```python
from build123d import *

# Parameters (mm, degrees)
F0_W     = 30.48
F0_H     = 28
F1_DEPTH = 1
F3_W     = 30.48
F3_H     = 4.265539
F4_DEPTH = 0.5
F2_R     = 0.9
F2_R_2   = 0.7
F2_R_3   = 0.65
F5_DEPTH = 2


with BuildPart() as f1:
    # F0 (on Top) → F1 (new body)
    with BuildSketch(Plane.XY):
        Rectangle(F0_W, F0_H)
    extrude(amount=F1_DEPTH)

    # F3 (on face) → F4 (cut)
    with BuildSketch(Plane.XY.offset(1)):
        with Locations((0, 1.480549)):
            Rectangle(F3_W, F3_H)
    extrude(amount=-F4_DEPTH, mode=Mode.SUBTRACT)

    # F2 (on face) → F5 (cut)
    with BuildSketch(Plane.XY.offset(1)):
        with Locations((-11.36, 11.94)):
            Circle(F2_R)
        with Locations((-6.28, 11.94)):
            Circle(F2_R)
        with Locations((-1.2, 11.94)):
            Circle(F2_R)
        with Locations((8.96, 11.94)):
            Circle(F2_R)
        with Locations((14.04, 11.94)):
            Circle(F2_R)
        with Locations((-11.36, 6.86)):
            Circle(F2_R)
        with Locations((-6.28, 6.86)):
            Circle(F2_R)
        with Locations((-1.2, 6.86)):
            Circle(F2_R)
        with Locations((8.96, 6.86)):
            Circle(F2_R)
        with Locations((14.04, 6.86)):
            Circle(F2_R)
        with Locations((-11.36, -9.52)):
            Circle(F2_R_2)
        with Locations((-6.28, -9.52)):
            Circle(F2_R_2)
        with Locations((-1.2, -9.52)):
            Circle(F2_R_2)
        with Locations((8.96, -9.52)):
            Circle(F2_R_2)
        with Locations((14.04, -9.52)):
            Circle(F2_R_2)
        with Locations((-11.36, -13.3)):
            Circle(F2_R_3)
        with Locations((-6.28, -13.3)):
            Circle(F2_R_3)
        with Locations((-1.2, -13.3)):
            Circle(F2_R_3)
        with Locations((8.96, -13.3)):
            Circle(F2_R_3)
        with Locations((14.04, -13.3)):
            Circle(F2_R_3)
    extrude(amount=-F5_DEPTH, mode=Mode.SUBTRACT)


solid = f1.part
```
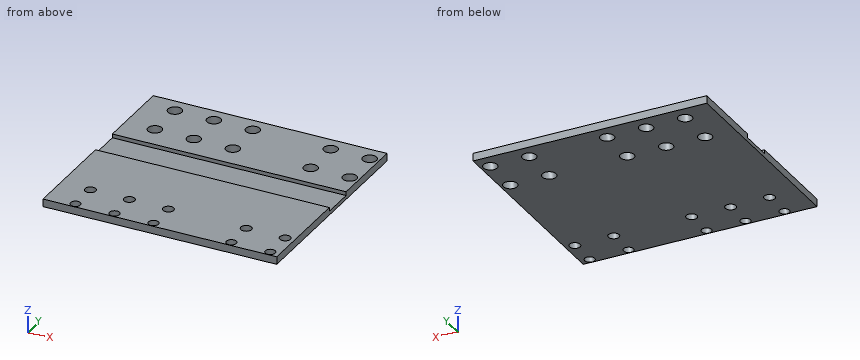
Geometry: final body of the model. Coordinates: model frame, mm. Coordinates: 2 decimals unless noted, no trailing zeros. Loops run counter-clockwise (first coordinate to the right, second up) from the corner with the lowest first, then second, coordinate; pieces in that order, holes last. Notation, with made-up numbers: (-23.5, 34) -> (9.5, 34) arc R22 ccw to (9.5, 45) -> close; hole circle Ø6 at (-6.5, 54). An arc over 180 degrees is marked (long way). Use a Markdown table: item, result. Add a question column.
(1) Section query C-C, the plane z = 0.8. State how many separate pieces and enclosed holes the cut face has, plus the area to 3 significant figures.
(2) Section query A-A, the plane x = -6.28. Return loops of the section in (y, z).
(3) Section query B-B, the plane y = -9.52. Return loops of the section in (x, z), plus the area to 3 significant figures.
(4) Line query: line 1 along X through (y, z) = (6.75, 0.15); line 2 along Z through (x, y) = (-7.5, 3.5); line 3 along X through (y, z) = (6.5, 0.9). Output: solid intervals per line, ascending.
(5) Section query D-D, the plane y = 6.86. Return loops of the section in (x, z).
Answer:
| question | item | result |
|---|---|---|
| 1 | separate pieces | 2 |
| 1 | enclosed holes | 20 |
| 1 | area | 684 mm^2 |
| 2 | outline | (-14, 0) -> (-13.95, 0) -> (-13.95, 1) -> (-14, 1) -> close; (-12.65, 0) -> (-10.22, 0) -> (-10.22, 1) -> (-12.65, 1) -> close; (-8.82, 0) -> (5.96, 0) -> (5.96, 1) -> (3.61, 1) -> (3.61, 0.5) -> (-0.65, 0.5) -> (-0.65, 1) -> (-8.82, 1) -> close; (7.76, 0) -> (11.04, 0) -> (11.04, 1) -> (7.76, 1) -> close; (12.84, 0) -> (14, 0) -> (14, 1) -> (12.84, 1) -> close |
| 3 | outline | (-15.24, 0) -> (-12.06, 0) -> (-12.06, 1) -> (-15.24, 1) -> close; (-10.66, 0) -> (-6.98, 0) -> (-6.98, 1) -> (-10.66, 1) -> close; (-5.58, 0) -> (-1.9, 0) -> (-1.9, 1) -> (-5.58, 1) -> close; (-0.5, 0) -> (8.26, 0) -> (8.26, 1) -> (-0.5, 1) -> close; (9.66, 0) -> (13.34, 0) -> (13.34, 1) -> (9.66, 1) -> close; (14.74, 0) -> (15.24, 0) -> (15.24, 1) -> (14.74, 1) -> close |
| 3 | area | 23.5 mm^2 |
| 4 | line 1 | x = -15.24 to -12.25, -10.47 to -7.17, -5.39 to -2.09, -0.31 to 8.07, 9.85 to 13.15, 14.93 to 15.24 |
| 4 | line 2 | z = 0 to 0.5 |
| 4 | line 3 | x = -15.24 to -12.18, -10.54 to -7.1, -5.46 to -2.02, -0.38 to 8.14, 9.78 to 13.22, 14.86 to 15.24 |
| 5 | outline | (-15.24, 0) -> (-12.26, 0) -> (-12.26, 1) -> (-15.24, 1) -> close; (-10.46, 0) -> (-7.18, 0) -> (-7.18, 1) -> (-10.46, 1) -> close; (-5.38, 0) -> (-2.1, 0) -> (-2.1, 1) -> (-5.38, 1) -> close; (-0.3, 0) -> (8.06, 0) -> (8.06, 1) -> (-0.3, 1) -> close; (9.86, 0) -> (13.14, 0) -> (13.14, 1) -> (9.86, 1) -> close; (14.94, 0) -> (15.24, 0) -> (15.24, 1) -> (14.94, 1) -> close |
